Can you work these out from the model? Positions are in its coordinate system, mm. Face numbers are marked on the shaded views. A direction names the side the tool comes from. Coordinates: 2 decimals unless noted, no trailing zeros. Order: outer loops, then holes, each group sorted by start corner. A loop starts at its lowest first (then second) coordinate and runs counter-clockwise, first axis right, second up. Notation, with made-up numbers: (60, 37.5) -> (110, 37.5) arc R10 ccw to (110, 43.5) -> close; hole circle Ø1 at (40, 18). An arc over 180 degrees is marked (long way). Answer in a Markdown table with one row per item. Add a question column.
1. Will these pins go through, and if not, where does the flat tip stop? pin 1 (20.5 mm diameter, centred on x = 38.1, z = 12.7, fed in from -Y); pin 2 (1.5 mm diameter, centred on y = -44.5, z = -8.5, fed in from -X); pin 3 (20.5 mm diameter, centred on x = -2.5, z = 3.5, fed in from +Y).
2. Imagine slicing it at C-C on x = -38.1. Write out the boundary of the cut face in (y, z), plus the area to 3 significant figures.
3. If I drill on line 1 along Z through (x, y) = (38, -9); line 2 along Z through (x, y) = (0, -37); line 3 along Y through (x, z) = (12.5, 0.5), over which ranges is the centre line in solid material (lowest first)? Write a range as [from, to].
4. Imagine slicing it at D-D on z = 0. Write out the boundary of the cut face in (x, y), plus the area to 3 significant figures.
5. Imagine slicing it at B-B on y = -13.5. Write out the boundary of the cut face in (x, z), plus the area to 3 significant figures.
6. Imagine slicing it at A-A on x = 0. Write out the boundary of the cut face in (y, z).
7. We'd pull the mould along X, two halves only. Please class the marked faces 1, 2 and 3: pulls with the +X half, pulls with the -X half, needs draft (parallel to the pull), parting line crosses it, or undercut.
8. On a 3-axis mill with a long thin cutter (end or side, diameter ignored), from which of +Z, -Z, +X, -X, +Y, -Y can I reach the whole of each face in a straight line? I mean the marked faces 4 and 5. Say none if no direction works.
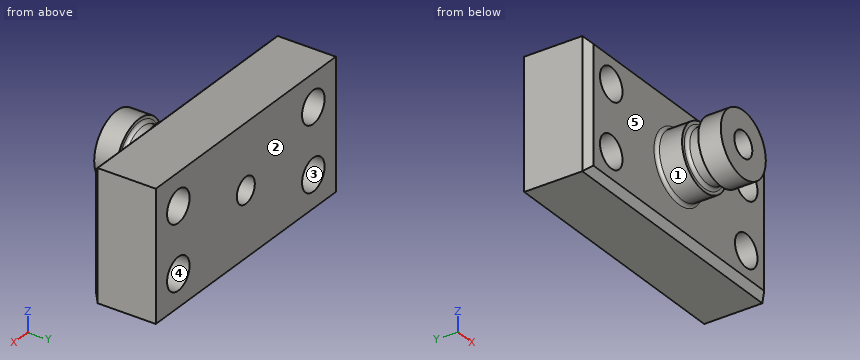
from build123d import *

# Parameters (mm, degrees)
F0_W      = 101.6
F0_H      = 50.8
F1_DEPTH  = 25.4
F2_R      = 6.35
F3_DEPTH  = 25.401
F4_W      = 12.7
F4_H      = 25.4
F6_W      = 14.885251
F6_H      = 6.35
F8_R      = 1.27
F9_SIZE   = 2.54
F10_R     = 5.08
F11_DEPTH = 50.801


with BuildPart() as f1:
    # F0 (on Front) → F1 (new body)
    with BuildSketch(Plane.XZ):
        Rectangle(F0_W, F0_H)
    extrude(amount=F1_DEPTH)

    # F2 (on face) → F3 (cut, through all)
    with BuildSketch(Plane.XZ.offset(25.4)):
        with Locations((-38.1, 12.7)):
            Circle(F2_R)
        with Locations((38.1, 12.7)):
            Circle(F2_R)
        with Locations((38.1, -12.7)):
            Circle(F2_R)
        with Locations((-38.1, -12.7)):
            Circle(F2_R)
    extrude(amount=-F3_DEPTH, mode=Mode.SUBTRACT)

    # F4 (on Top) → F5 (revolve)
    with BuildSketch(Plane.XY):
        with Locations((6.35, -38.1)):
            Rectangle(F4_W, F4_H)
    revolve(axis=Axis((0, -38.1, 0), (0, -1, 0)))

    # F6 (on Top) → F7 (revolve, cut)
    with BuildSketch(Plane.XY):
        with Locations((-17.602626, -38.735)):
            Rectangle(F6_W, F6_H)
    revolve(axis=Axis((0, -35.056077, 0), (0, 1, 0)), mode=Mode.SUBTRACT)

    # F8
    f8_edges = [f1.edges().sort_by_distance(p)[0] for p in [
        (-12.7, -25.4, 0),
        (10.16, -35.56, 0),
        (10.16, -41.91, 0),
    ]]
    fillet(f8_edges, radius=F8_R)

    # F9
    f9_edges = [f1.edges().sort_by_distance(p)[0] for p in [
        (0, -25.4, -25.4),
        (0, -25.4, 25.4),
        (50.8, -25.4, 0),
        (-50.8, -25.4, 0),
    ]]
    chamfer(f9_edges, length=F9_SIZE)

    # F10 (on face) → F11 (cut, through all)
    with BuildSketch(Plane.XZ.offset(50.8)):
        Circle(F10_R)
    extrude(amount=-F11_DEPTH, mode=Mode.SUBTRACT)


solid = f1.part
Answers follow:
| question | item | result |
|---|---|---|
| 1 | pin 1 | stops at y = -25.4 |
| 1 | pin 2 | stops at x = -10.06 |
| 1 | pin 3 | stops at y = 0 |
| 2 | outline | (-25.4, -22.86) -> (-22.86, -25.4) -> (0, -25.4) -> (0, -19.05) -> (-25.4, -19.05) -> close; (-25.4, -6.35) -> (0, -6.35) -> (0, 6.35) -> (-25.4, 6.35) -> close; (-25.4, 19.05) -> (0, 19.05) -> (0, 25.4) -> (-22.86, 25.4) -> (-25.4, 22.86) -> close |
| 2 | area | 639 mm² |
| 3 | line 1 | z = [-25.4, -19.05], [-6.35, 6.35], [19.05, 25.4] |
| 3 | line 2 | z = [-10.16, -5.08], [5.08, 10.16] |
| 3 | line 3 | y = [-50.8, -41.91], [-35.56, 0] |
| 4 | outline | (-50.8, -22.86) -> (-48.26, -25.4) -> (-13.97, -25.4) arc R1.27 cw to (-12.7, -26.67) -> (-12.7, -35.56) -> (-11.43, -35.56) arc R1.27 cw to (-10.16, -36.83) -> (-10.16, -40.64) arc R1.27 cw to (-11.43, -41.91) -> (-12.7, -41.91) -> (-12.7, -50.8) -> (-5.08, -50.8) -> (-5.08, 0) -> (-50.8, 0) -> close; (5.08, -50.8) -> (12.7, -50.8) -> (12.7, -41.91) -> (11.43, -41.91) arc R1.27 cw to (10.16, -40.64) -> (10.16, -36.83) arc R1.27 cw to (11.43, -35.56) -> (12.7, -35.56) -> (12.7, -26.67) arc R1.27 cw to (13.97, -25.4) -> (48.26, -25.4) -> (50.8, -22.86) -> (50.8, 0) -> (5.08, 0) -> close |
| 4 | area | 2,670 mm² |
| 5 | outline | (-50.8, -25.4) -> (50.8, -25.4) -> (50.8, 25.4) -> (-50.8, 25.4) -> close; hole circle Ø12.7 at (-38.1, -12.7); hole circle Ø12.7 at (-38.1, 12.7); hole circle Ø10.16 at (0, 0); hole circle Ø12.7 at (38.1, -12.7); hole circle Ø12.7 at (38.1, 12.7) |
| 5 | area | 4,570 mm² |
| 6 | outline | (-50.8, -12.7) -> (-41.91, -12.7) -> (-41.91, -11.43) arc R1.27 cw to (-40.64, -10.16) -> (-36.83, -10.16) arc R1.27 cw to (-35.56, -11.43) -> (-35.56, -12.7) -> (-26.67, -12.7) arc R1.27 cw to (-25.4, -13.97) -> (-25.4, -22.86) -> (-22.86, -25.4) -> (0, -25.4) -> (0, -5.08) -> (-50.8, -5.08) -> close; (-50.8, 5.08) -> (0, 5.08) -> (0, 25.4) -> (-22.86, 25.4) -> (-25.4, 22.86) -> (-25.4, 13.97) arc R1.27 cw to (-26.67, 12.7) -> (-35.56, 12.7) -> (-35.56, 11.43) arc R1.27 cw to (-36.83, 10.16) -> (-40.64, 10.16) arc R1.27 cw to (-41.91, 11.43) -> (-41.91, 12.7) -> (-50.8, 12.7) -> close |
| 7 | face 1 | parting line crosses it |
| 7 | face 2 | needs draft |
| 7 | face 3 | undercut |
| 8 | face 4 | +Y, -Y |
| 8 | face 5 | -Y |
